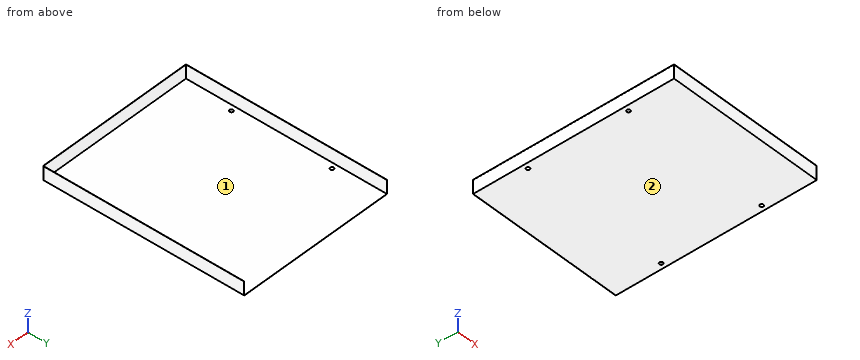
```python
from build123d import *

# Parameters (mm, degrees)
SKETCH1_W             = 89.6514
SKETCH1_H             = 226.9314
SKETCH1_R             = 2
HEAT_EXCHANGER_DEPTH  = 0.0686
CONVECTION_FINS_DEPTH = 15.29686
TOP_OVERWRAP_DEPTH    = 0.0686
SIDE_OVERWRAP_DEPTH   = 0.0686


# Read off the part's stored shape, not the designer's step: Mirror1
with BuildPart() as part:
    # Sketch1 → Heat Exchanger (new body)
    with BuildSketch(Plane.XY):
        with Locations((-44.8257, 0)):
            Rectangle(SKETCH1_W, SKETCH1_H)
        with Locations((-83.71996294, -56.7081132)):
            Circle(SKETCH1_R, mode=Mode.SUBTRACT)
        with Locations((-83.71996294, 56.94427919)):
            Circle(SKETCH1_R, mode=Mode.SUBTRACT)
    extrude(amount=HEAT_EXCHANGER_DEPTH)

    # Sketch3 → Convection Fins (add)
    with BuildSketch(Plane.XY):
        Polygon((0, -113.5343), (0, -113.4657), (-89.6514, -113.4657), (-89.6514, 113.4657), (-89.72, 113.4657), (-89.72, -113.5343), align=None)
    extrude(amount=CONVECTION_FINS_DEPTH)

    # Sketch5 → Top Overwrap (add)
    with BuildSketch(Plane(origin=(0, 113.4657, 0), x_dir=(1, 0, 0), z_dir=(0, 1, 0))):
        Polygon((-89.8724, -15.29686), (-89.6514, -15.29686), (-89.6514, -0.0686), (0, -0.0686), (0, 0.1524), (-89.8724, 0.1524), align=None)
    extrude(amount=TOP_OVERWRAP_DEPTH)

    # Sketch7 → Side Overwrap (add)
    with BuildSketch(Plane.XY.offset(15.29686)):
        Polygon((-89.8724, 113.5343), (-89.6514, 113.5343), (-89.6514, -113.4657), (0, -113.4657), (0, -113.6867), (-89.8724, -113.6867), align=None)
    extrude(amount=SIDE_OVERWRAP_DEPTH)

    # Mirror1: part across plane


with BuildPart() as part_1:
    add(part.part)
    add(part.part.mirror(Plane(origin=(0, 0, 0), x_dir=(0, 0, 1), z_dir=(1, 0, 0))))


solid = part_1.part
```
Read the model definition and answer for the solid it produces. Units are mm, in the model's axes. Face numbers are marked on the shaded views. Coordinates: 2 decimals unless noted, no trailing zeros. Write each loop counter-clockwise with the first axis right and the second up, starting at its lowest first coordinate (ties: lowest second). Pieces come first, ordered by that corner, then holes. Notation, with made-up numbers: (-2.5, 6) -> (11.5, 6) arc R13 ccw to (11.5, 15) -> close; hole circle Ø8 at (76.25, -25.75). An arc over 180 degrees is marked (long way). Write item = value, one per line.
(1) For a pull along X with two mould halves and no side action, classify the marked faces 1 and 2 as +X half, -X half, draft (parallel to the pull), parting line (faces both ways), or undercut.
From the geometry:
face_1 = undercut
face_2 = draft
(2) Section C-C on z = 12.5 is taken. Write down the section's boundary in (x, y).
From the geometry:
outline = (-89.87, 113.47) -> (-89.72, 113.47) -> (-89.72, -113.53) -> (89.72, -113.53) -> (89.72, 113.47) -> (89.87, 113.47) -> (89.87, 113.53) -> (89.65, 113.53) -> (89.65, -113.47) -> (-89.65, -113.47) -> (-89.65, 113.53) -> (-89.87, 113.53) -> close
(3) Section B-B on x = -77.5 is taken. Write down the section's boundary in (y, z).
From the geometry:
outline = (-113.69, 15.3) -> (-113.53, 15.3) -> (-113.53, 0) -> (113.47, 0) -> (113.47, -0.15) -> (113.53, -0.15) -> (113.53, 0.07) -> (-113.47, 0.07) -> (-113.47, 15.37) -> (-113.69, 15.37) -> close
(4) Section A-A on y = 34.5 is taken. Write down the section's boundary in (x, z).
From the geometry:
outline = (-89.87, 15.3) -> (-89.72, 15.3) -> (-89.72, 0) -> (89.72, 0) -> (89.72, 15.3) -> (89.87, 15.3) -> (89.87, 15.37) -> (89.65, 15.37) -> (89.65, 0.07) -> (-89.65, 0.07) -> (-89.65, 15.37) -> (-89.87, 15.37) -> close
(5) Given pin 1 Ø3 at (x, y) = (83.72, -56.71) entering from +Z; pin 2 Ø6 at (x, y) = (1.5, 54.5) entering from +Z; pin 3 Ø3 at (x, y) = (58, 24) entering from -Z; pin 4 Ø6 at (y, z) = (-44, 4.5) entering from +X, each flat-ended and moving along its own axis, determine where each tip first touches the part or whether it passes through.
From the geometry:
pin_1 = through
pin_2 = 0.07
pin_3 = 0
pin_4 = 89.72
